from build123d import *

# Parameters (mm, degrees)
SKETCH1_R               = 6.8
SKETCH1_R_2             = 5.3
BOSS_EXTRUDE1_DEPTH     = 5.8
SKETCH2_R               = 6.8
BOSS_EXTRUDE2_DEPTH     = 2.2
FILLET1_R               = 2
SKETCH4_W               = 5
SKETCH4_H               = 4.2
CUT_EXTRUDE1_DEPTH      = 13.509196726
CUT_EXTRUDE2_DEPTH      = 13.509196726
CUT_EXTRUDE2_DEPTH_BACK = 13.509196726
SKETCH5_W               = 1.5
SKETCH5_H               = 5.8
SKETCH3_R               = 3
BOSS_EXTRUDE3_DEPTH     = 2.5


with BuildPart() as part:
    # Sketch1 → Boss-Extrude1 (new body)
    with BuildSketch(Plane(origin=(0, 0, 0), x_dir=(1, 0, 0), z_dir=(0, 1, 0))):
        with Locations(Location((0, 0, 0), (0, 0, 270))):
            Circle(SKETCH1_R)
        with Locations(Location((0, 0, 0), (0, 0, 270))):
            Circle(SKETCH1_R_2, mode=Mode.SUBTRACT)
    extrude(amount=BOSS_EXTRUDE1_DEPTH)

    # Sketch2 → Boss-Extrude2 (add)
    with BuildSketch(Plane(origin=(0, 5.8, 0), x_dir=(1, 0, 0), z_dir=(0, 1, 0))):
        with Locations(Location((0, 0, 0), (0, 0, 270))):
            Circle(SKETCH2_R)
    extrude(amount=BOSS_EXTRUDE2_DEPTH)

    # Fillet1
    fillet1_edges = [part.edges().sort_by_distance(p)[0] for p in [
        (0, 8, -6.8),
    ]]
    fillet(fillet1_edges, radius=FILLET1_R)

    # Sketch4 → Cut-Extrude1 (cut, through all)
    with BuildSketch(Plane.XY):
        with Locations((0, 2.1)):
            Rectangle(SKETCH4_W, SKETCH4_H)
    extrude(amount=CUT_EXTRUDE1_DEPTH, mode=Mode.SUBTRACT)

    # Sketch5 → Cut-Extrude2 (cut, two sides: drawn at the far end of the back side and taken through both)
    with BuildSketch(Plane(origin=(0, 0, 0), x_dir=(0, 0, -1), z_dir=(1, 0, 0)).offset(-CUT_EXTRUDE2_DEPTH_BACK)):
        with Locations((0, 2.9)):
            Rectangle(SKETCH5_W, SKETCH5_H)
    extrude(amount=CUT_EXTRUDE2_DEPTH + CUT_EXTRUDE2_DEPTH_BACK, mode=Mode.SUBTRACT)

    # Sketch3 → Boss-Extrude3 (add)
    with BuildSketch(Plane.XZ.offset(-5.8)):
        with Locations(Location((0, 0, 0), (0, 0, 90))):
            Circle(SKETCH3_R)
    extrude(amount=BOSS_EXTRUDE3_DEPTH)


solid = part.part
Read the model definition and answer for the solid it produces. Units are mm, in the model's axes. A direction names the side the tool comes from. Round coordinates to 2 decimals unless told otherwise and drop trailing zeros. Loops run counter-clockwise (first coordinate to the right, second up) from the corner with the lowest first, then second, coordinate; pieces in that order, holes last. Notation, with made-up numbers: (-12.75, 6.25) - (37.25, 6.25) arc R9 ccw to (37.25, 20.25) - close; hole circle Ø8 at (68, 78). An arc over 180 degrees is marked (long way). One line per question, with ' | ' between items. Start each with the question number.
Q1. Find the intervals of material crossed by L1, parallel to Y at x = 3.75, z = 2.5; L2, parallel to Z at x = 5.75, y = 5; L3, parallel to X at y = 4, z = 6, in increasing order.
Q2. For a pull along Z with two mould halves and no side action, classify faces 4 (the flat face through (6, 3, -0.75)), 5 (the cylindrical face through (-4.138, 2.958, -5.396)), 6 (the flat face through (2.5, 2, 5)) as +Z half, -Z half, draft (parallel to the pull), parting line (faces both ways), or undercut.
Q3. Section B-B on x = 0 is taken. Give the vertices of the cut face in (y, z), plus the area to 3 significant figures.
Q4. For faces 1 (the flat face through (0, 4.2, 6)), 2 (the flat face through (6, 3, 0.75)), 3 (the flat face through (-6, 3, 0.75)), determine the directions among +Z, -Z, +X, -X, +Y, -Y from which every point of the face is accessible in a straight line to the end or side of a thin tool.
Q5. Section A-A on y = 1 is taken. Give the vertices of the cut face in (x, z).
Q6. Flat-ended cylindrical pins translate along their axes: pin 1 (1.8 mm diameter, centred on y = 2.5, z = 5, fed in from -X); pin 2 (2 mm diameter, centred on x = -4.5, y = 2, fed in from +Z); pin 3 (2.5 mm diameter, centred on x = 1, z = 6, fed in from -Y). Find the tip coordinate at first contact, or state that the pin passes through.
Q7. Section C-C on z = 0 is taken. Give the vertices of the cut face in (x, y).
Established:
1) L1: 5.8 to 8 | L2: -3.63 to -0.75, 0.75 to 3.63 | L3: -3.2 to -2.5, 2.5 to 3.2
2) face 4: undercut | face 5: parting line | face 6: draft
3) outline: (0, -6.8) - (6, -6.8) arc R2 ccw to (8, -4.8) - (8, 4.8) arc R2 ccw to (6, 6.8) - (4.2, 6.8) - (4.2, 5.3) - (5.8, 5.3) - (5.8, 3) - (3.3, 3) - (3.3, -3) - (5.8, -3) - (5.8, -5.3) - (0, -5.3) - close | area: 54.3 mm²
4) face 1: +Z, -Y | face 2: +X, -Y | face 3: -X, -Y
5) outline: (-6.76, -0.75) arc R6.8 ccw to (6.76, -0.75) - (5.25, -0.75) arc R5.3 cw to (-5.25, -0.75) - close; (-6.76, 0.75) - (-5.25, 0.75) arc R5.3 cw to (-2.5, 4.67) - (-2.5, 6.32) arc R6.8 ccw to start; (2.5, 4.67) arc R5.3 cw to (5.25, 0.75) - (6.76, 0.75) arc R6.8 ccw to (2.5, 6.32) - close
6) pin 1: x = -5.42 | pin 2: z = 5.83 | pin 3: y = 4.2
7) outline: (-6.8, 5.8) - (-3, 5.8) - (-3, 3.3) - (3, 3.3) - (3, 5.8) - (6.8, 5.8) - (6.8, 6) arc R2 ccw to (4.8, 8) - (-4.8, 8) arc R2 ccw to (-6.8, 6) - close
